from build123d import *

# Parameters (mm, degrees)
SKETCH_1_W           = 30
SKETCH_1_H           = 48
EXTRUDE_1_DEPTH      = 3
SKETCH_3_W           = 30
SKETCH_3_H           = 3
EXTRUDE_2_DEPTH      = 35
CUT_EXTRUDE_2_DEPTH  = 69.176242196
CUT_EXTRUDE_3_DEPTH  = 69.176242196
SKETCH_7_W           = 3
SKETCH_7_H           = 42
EXTRUDE_3_DEPTH      = 25
SKETCH_14_W          = 3
SKETCH_14_H          = 42
EXTRUDE_6_DEPTH      = 30
SKETCH_15_R          = 1.65
CUT_EXTRUDE_6_DEPTH  = 4
SKETCH_16_R          = 1.15
SKETCH_16_W          = 12.5
SKETCH_16_H          = 23
CUT_EXTRUDE_7_DEPTH  = 10
SKETCH_17_W          = 30.8
SKETCH_17_H          = 5
CUT_EXTRUDE_8_DEPTH  = 10
SKETCH_20_R          = 1.5
CUT_EXTRUDE_11_DEPTH = 82.043198357
CUT_EXTRUDE_12_REACH = 83.043
SKETCH_22_R          = 2
SKETCH_23_W          = 5.554421841
SKETCH_23_H          = 4.674351411
SKETCH_23_R          = 2
EXTRUDE_9_DEPTH      = 3


with BuildPart() as part:
    # 草图1 → 凸台-拉伸1 (new body)
    with BuildSketch(Plane.XY):
        with Locations((15, 24)):
            Rectangle(SKETCH_1_W, SKETCH_1_H)
    extrude(amount=EXTRUDE_1_DEPTH)

    # 草图3 → 凸台-拉伸2 (add)
    with BuildSketch(Plane.XY.offset(3)):
        with Locations((15, 46.5)):
            Rectangle(SKETCH_3_W, SKETCH_3_H)
        with Locations((15, 1.5)):
            Rectangle(SKETCH_3_W, SKETCH_3_H)
    extrude(amount=EXTRUDE_2_DEPTH)

    # 草图5 → 切除-拉伸2 (cut, through all)
    with BuildSketch(Plane.XZ):
        Polygon((0, 33), (5, 38), (0, 38), align=None)
    extrude(amount=-CUT_EXTRUDE_2_DEPTH, mode=Mode.SUBTRACT)

    # 草图6 → 切除-拉伸3 (cut, through all)
    with BuildSketch(Plane.XZ):
        Polygon((20, 0), (30, 10), (30, 0), align=None)
    extrude(amount=-CUT_EXTRUDE_3_DEPTH, mode=Mode.SUBTRACT)

    # 草图7 → 凸台-拉伸3 (add)
    with BuildSketch(Plane.XY.offset(3)):
        with Locations((1.5, 24)):
            Rectangle(SKETCH_7_W, SKETCH_7_H)
    extrude(amount=EXTRUDE_3_DEPTH)

    # 草图14 → 凸台-拉伸6 (add)
    with BuildSketch(Plane.XY.offset(28)):
        with Locations((1.5, 24)):
            Rectangle(SKETCH_14_W, SKETCH_14_H)
    extrude(amount=EXTRUDE_6_DEPTH)

    # 草图15 → 切除-拉伸6 (cut)
    with BuildSketch(Plane.ZY):
        with Locations(Location((38, 13, 0), (0, 0, 270))):
            Circle(SKETCH_15_R)
        with Locations(Location((38, 38, 0), (0, 0, 270))):
            Circle(SKETCH_15_R)
        with Locations(Location((53, 38, 0), (0, 0, 270))):
            Circle(SKETCH_15_R)
        with Locations(Location((53, 13, 0), (0, 0, 270))):
            Circle(SKETCH_15_R)
    extrude(amount=-CUT_EXTRUDE_6_DEPTH, mode=Mode.SUBTRACT)

    # 草图16 → 切除-拉伸7 (cut)
    with BuildSketch(Plane.XY.offset(3)):
        with Locations((9.25, 32.85)):
            Circle(SKETCH_16_R)
        with Locations((9.25, 5.15)):
            Circle(SKETCH_16_R)
        with Locations((9.25, 19)):
            Rectangle(SKETCH_16_W, SKETCH_16_H)
    extrude(amount=-CUT_EXTRUDE_7_DEPTH, mode=Mode.SUBTRACT)

    # 草图17 → 切除-拉伸8 (cut)
    with BuildSketch(Plane.ZY):
        with Locations((42.6, 5.5)):
            Rectangle(SKETCH_17_W, SKETCH_17_H)
    extrude(amount=-CUT_EXTRUDE_8_DEPTH, mode=Mode.SUBTRACT)

    # 草图20 → 切除-拉伸11 (cut, through all)
    with BuildSketch(Plane.XZ):
        with Locations(Location((26.5, 34.5, 0), (0, 0, 270))):
            Circle(SKETCH_20_R)
        with Locations(Location((11.5, 34.5, 0), (0, 0, 270))):
            Circle(SKETCH_20_R)
    extrude(amount=-CUT_EXTRUDE_11_DEPTH, mode=Mode.SUBTRACT)

    # 草图22 → 切除-拉伸12 (cut, up to next)
    with BuildSketch(Plane(origin=(0, 0, 0), x_dir=(-1, 0, 0), z_dir=(0, 0, -1)), mode=Mode.PRIVATE) as cut_extrude_12_sk1:
        with Locations((-9.25, 37.75)):
            Circle(SKETCH_22_R)
    cut_extrude_12_tool1 = extrude(cut_extrude_12_sk1.sketch, amount=-CUT_EXTRUDE_12_REACH, mode=Mode.PRIVATE) & part.part
    add(cut_extrude_12_tool1.solids().sort_by_distance((9.25, 37.75, 0))[0], mode=Mode.SUBTRACT)

    # 草图23 → 凸台-拉伸9 (add)
    with BuildSketch(Plane.XY.offset(3)):
        with Locations((9.150966926, 37.89409872)):
            Rectangle(SKETCH_23_W, SKETCH_23_H)
        with Locations(Location((9.25, 37.75, 0), (0, 0, 180))):
            Circle(SKETCH_23_R, mode=Mode.SUBTRACT)
    extrude(amount=EXTRUDE_9_DEPTH)


solid = part.part
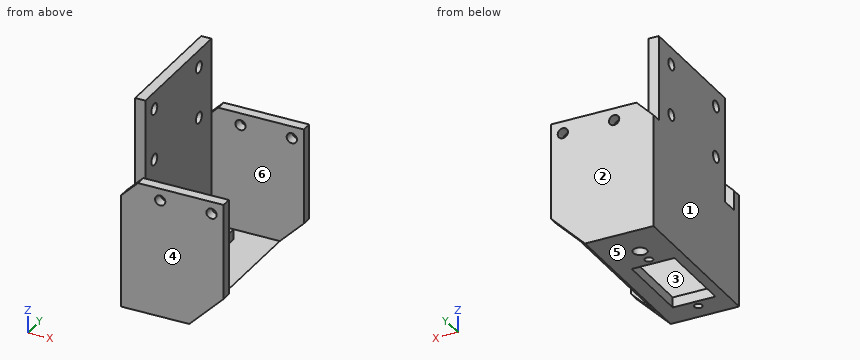
Work out the finished part from the listing and answer in its coordinate system (mm). Face numbers are marked on the shaded views. A direction names the side the tool comes from. Round coordinates to 2 decimals unless told otherwise and drop trailing zeros. Loops run counter-clockwise (first coordinate to the right, second up) from the corner with the lowest first, then second, coordinate; pieces in that order, holes last. Notation, with made-up numbers: (14.25, -28.5) -> (65.25, -28.5) arc R15 ccw to (65.25, -4.5) -> close; hole circle Ø11 at (63, -13). An arc over 180 degrees is marked (long way). Use one line per item in the form item = value.
(1) Find section B-B on z = 53. Give the vertices of the cut face in (x, y), then the cut area to 3 significant figures.
Answer list:
outline = (0, 8) -> (3, 8) -> (3, 11.35) -> (0, 11.35) -> close; (0, 14.65) -> (3, 14.65) -> (3, 36.35) -> (0, 36.35) -> close; (0, 39.65) -> (3, 39.65) -> (3, 45) -> (0, 45) -> close
area = 91.2 mm2
(2) Find section D-D on x = 9.25. Give the vertices of the cut face in (y, z).
Answer list:
outline = (0, 0) -> (4, 0) -> (4, 3) -> (3, 3) -> (3, 38) -> (0, 38) -> close; (6.3, 0) -> (7.5, 0) -> (7.5, 3) -> (6.3, 3) -> close; (30.5, 0) -> (31.7, 0) -> (31.7, 3) -> (30.5, 3) -> close; (34, 0) -> (35.75, 0) -> (35.75, 6) -> (35.56, 6) -> (35.56, 3) -> (34, 3) -> close; (39.75, 0) -> (48, 0) -> (48, 38) -> (45, 38) -> (45, 3) -> (40.23, 3) -> (40.23, 6) -> (39.75, 6) -> close
(3) A tool of negligible diameter and unlimited length cuts with its end or side. For the marked faces 5 and 6, from which of +Z, -Z, +X, -X, +Y, -Y can it reach the whole face along a straight path? Write none if from no direction.
Answer list:
face_5 = -Z, +X, -X, +Y, -Y
face_6 = +Z, +X
(4) Find section A-A on y = 5.15. Give the vertices of the cut face in (x, z), then the cut area to 3 significant figures.
Answer list:
outline = (0, 0) -> (8.1, 0) -> (8.1, 3) -> (3, 3) -> (3, 27.2) -> (0, 27.2) -> close; (10.4, 0) -> (20, 0) -> (23, 3) -> (10.4, 3) -> close
area = 130 mm2
(5) Find section C-C on x = 26.5. Give the vertices of the cut face in (y, z), then the cut area to 3 significant figures.
Answer list:
outline = (0, 6.5) -> (3, 6.5) -> (3, 33) -> (0, 33) -> close; (0, 36) -> (3, 36) -> (3, 38) -> (0, 38) -> close; (45, 6.5) -> (48, 6.5) -> (48, 33) -> (45, 33) -> close; (45, 36) -> (48, 36) -> (48, 38) -> (45, 38) -> close
area = 171 mm2
(6) For a pull along Y with two mould halves and no side action, classify the marked faces 1, 2, 3 and 4 as released by +Y, released by -Y, zero draft, split by the parting line, or undercut.
Answer list:
face_1 = zero draft
face_2 = released by +Y
face_3 = undercut
face_4 = released by -Y
(7) Flat-ended cylindrical pins translate along their axes: P1, Ø1.5, axis at y = 16, z = 20.5, coming from the +X side; P2, Ø1.5, axis at x = 19.5, y = 12, coming from the +Z side; P3, Ø0.9, axis at x = 1, y = 6.5, coming from the +Z side. Find the tip coordinate at first contact, or state that the pin passes through.
Answer list:
P1 = 3
P2 = 3
P3 = 27.2
(8) Straight lines are drawn through the part: line 1 (Y direction, x = 9.25, z = 1.75); line 2 (Z direction, x = 1.2, y = 13); line 3 (Y direction, x = 27.5, z = 13.5). For each, find the intervals that lie inside material, in ascending order.
Answer list:
line_1 = 0 to 4, 6.3 to 7.5, 30.5 to 31.7, 34 to 35.75, 39.75 to 48
line_2 = 0 to 36.35, 39.65 to 51.35, 54.65 to 58
line_3 = 0 to 3, 45 to 48
